from build123d import *

# Parameters (mm, degrees)
EXTRUDE_1_DEPTH     = 23.5
SKETCH_6_R          = 16
CUT_EXTRUDE_8_DEPTH = 22.5
SKETCH_7_R          = 12.5
CUT_EXTRUDE_9_DEPTH = 2


with BuildPart() as part:
    # Эскиз1 → Вытянуть1 (new body)
    with BuildSketch(Plane.XY):
        with BuildLine():
            Line((18.943049375, -11.187532363), (18.832657697, 11.372378998))
            ThreePointArc((18.832657697, 11.372378998), (-21.99973662, -0.107650593), (18.943049375, -11.187532363))
        make_face()
    extrude(amount=EXTRUDE_1_DEPTH)

    # Эскиз6 → Вытянуть8 (cut)
    with BuildSketch(Plane(origin=(0, 0, 0), x_dir=(-1, 0, 0), z_dir=(0, 0, -1))):
        Circle(SKETCH_6_R)
    extrude(amount=-CUT_EXTRUDE_8_DEPTH, mode=Mode.SUBTRACT)

    # Эскиз7 → Вытянуть9 (cut, through all)
    with BuildSketch(Plane(origin=(0, 0, 22.5), x_dir=(-1, 0, 0), z_dir=(0, 0, -1))):
        Circle(SKETCH_7_R)
    extrude(amount=-CUT_EXTRUDE_9_DEPTH, mode=Mode.SUBTRACT)


solid = part.part
Geometry: final body of the model. Coordinates: model frame, mm. Round coordinates to 2 decimals unless told otherwise and drop trailing zeros. Loops run counter-clockwise (first coordinate to the right, second up) from the corner with the lowest first, then second, coordinate; pieces in that order, holes last.
Q1. Pull-direction query (Y, two-part tool) for faces 1 (the cylindrical face through (-21.99, 0.69, 11.59)), 2 (the flat face through (10, -8, 22.5)), 3 (the cylindrical face through (3.47, -15.62, 11.09)), 4 (the flat face through (-15.5, 5.2, 0)); classes: released by +Y, released by -Y, zero draft, split by the parting line, or undercut.
Q2. Section C-C on z = 4.5. Return loops of the section in (x, y).
Q3. Section D-D on x = 14. Return loops of the section in (y, z), plus the area to 3 significant figures.
Q4. Material intervals for L1, parallel to Y at x = 0, z = 6; L2, parallel to X at y = -2.5, z = 2.5; L3, parallel to Z at x = 7.5, y = 14, sorted ascending.
Q5. Pin query (flat end, axial travel): P1, Ø8, axis at x = 14.5, z = 12.5, coming from the -Y side; P2, Ø3, axis at x = 15, z = 8, coming from the -Y side; P3, Ø1.5, axis at y = 15.5, z = 6, coming from the -X side. Return the tip coordinate at first contact, or that it passes through.
Q6. Section B-B on y = 0. Return loops of the section in (x, z), plus the area to 3 significant figures.
Q7. Section A-A on x = 0. Return loops of the section in (y, z), plus the area to 3 significant figures.
Evaluation:
1. face 1: split by the parting line
1. face 2: undercut
1. face 3: undercut
1. face 4: zero draft
2. outline: (18.83, 11.37) arc R22 ccw (long way) to (18.94, -11.19) - close; hole circle Ø32 at (0, 0)
3. outline: (-16.97, 0) - (-7.75, 0) - (-7.75, 22.5) - (7.75, 22.5) - (7.75, 0) - (16.97, 0) - (16.97, 23.5) - (-16.97, 23.5) - close
3. area: 449 mm2
4. L1: y = -22 to -16, 16 to 22
4. L2: x = -21.86 to -15.8, 15.8 to 18.9
4. L3: z = 22.5 to 23.5
5. P1: stops at y = -19.33
5. P2: stops at y = -17.37
5. P3: stops at x = -16.32
6. outline: (-22, 0) - (-16, 0) - (-16, 22.5) - (-12.5, 22.5) - (-12.5, 23.5) - (-22, 23.5) - close; (12.5, 22.5) - (16, 22.5) - (16, 0) - (18.89, 0) - (18.89, 23.5) - (12.5, 23.5) - close
6. area: 216 mm2
7. outline: (-22, 0) - (-16, 0) - (-16, 22.5) - (-12.5, 22.5) - (-12.5, 23.5) - (-22, 23.5) - close; (12.5, 22.5) - (16, 22.5) - (16, 0) - (22, 0) - (22, 23.5) - (12.5, 23.5) - close
7. area: 289 mm2
